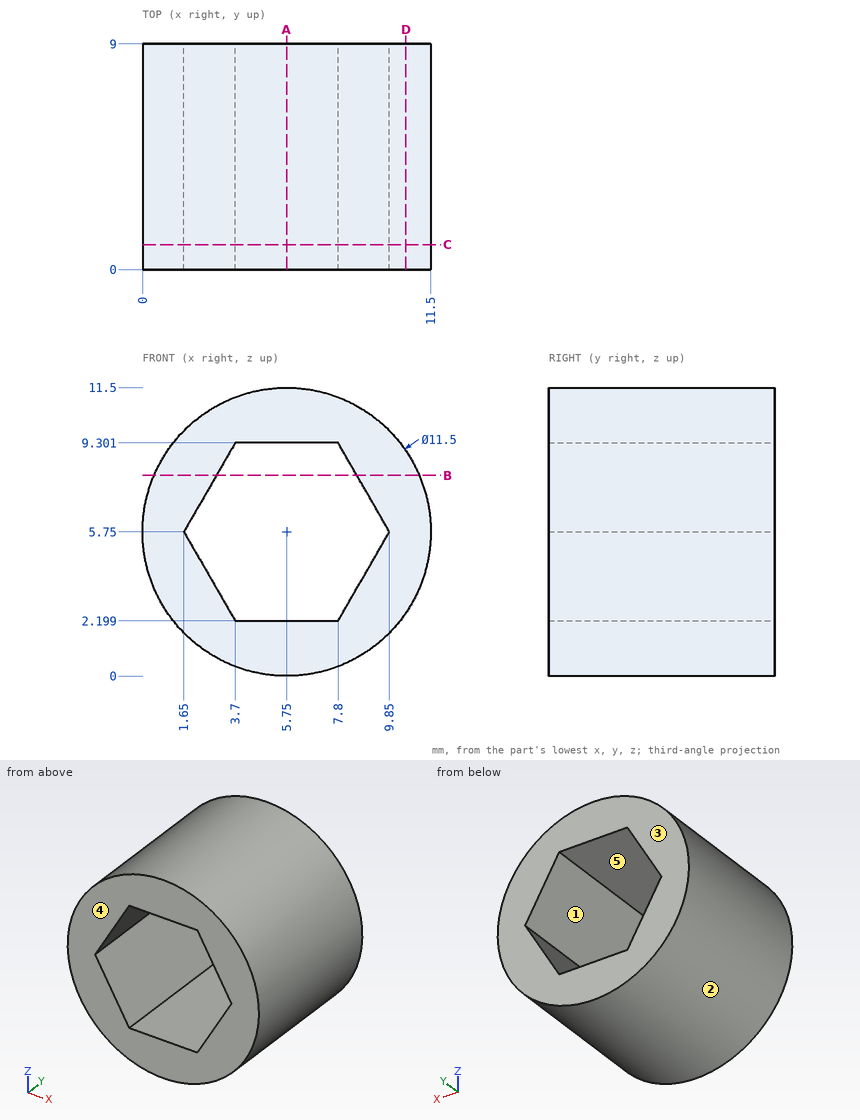
Study the drawing (mm; zero at the part's minimum x, y, z) and answer. A direction names the side the tool comes from. Round coordinates to 2 decimals unless told otherwise and drop trailing zeros. Write each loop counter-clockwise with the first axis right and the second up, starting at its lowest first coordinate (ties: lowest second). Pieces come first, ordered by that corner, then holes.
1) A cutting plane is placed at D-D (x = 10.5). Give the vertices of the cut face in (y, z).
2) Straight lines are drawn through the part: line 1 (Z direction, x = 6, y = 6.25) (1 decimal); line 2 (Z direction, x = 4, y = 4.25); line 3 (X direction, y = 5.5, z = 4.5). For each, find the intervals that lie inside material, in ascending order.
3) Given pin 1 Ø1.2 at (x, y) = (6.5, 2.5) entering from +Z; pin 2 Ø1.2 at (x, y) = (7, 4) entering from -Z; pin 3 Ø1 at (y, z) = (4, 1.5) entering from -X, each flat-ended and moving along its own axis, determine where each tip first touches the part or whether it passes through.
4) A tool of negligible diameter and unlimited length cuts with its end or side. For the marked faces 4 and 5, from which of +Z, -Z, +X, -X, +Y, -Y can it reach the whole face along a straight path? Write none if from no direction.
5) A cutting plane is placed at A-A (x = 5.75). Give the vertices of the cut face in (y, z), plus the area to 3 significant figures.
6) A cutting plane is placed at B-B (z = 8). Give the vertices of the cut face in (x, y).
7) A cutting plane is placed at C-C (y = 1). Give the vertices of the cut face in (x, z), plus the area to 3 significant figures.
8) The mould has two halves that part along Z. Classify the marked faces 1, 2 and 3: pulls with the +Z half, pulls with the -Z half, needs draft (parallel to the pull), parting line crosses it, or undercut.
Completed:
1. outline: (0, 2.51) - (9, 2.51) - (9, 8.99) - (0, 8.99) - close
2. line 1: z = 0 to 2.2, 9.3 to 11.5
2. line 2: z = 0.27 to 2.2, 9.3 to 11.23
2. line 3: x = 0.14 to 2.37, 9.13 to 11.36
3. pin 1: stops at z = 11.5
3. pin 2: stops at z = 0.04
3. pin 3: stops at x = 1.39
4. face 4: +Z, -Z, +X, -X, -Y
4. face 5: +Y, -Y
5. outline: (0, 0) - (9, 0) - (9, 2.2) - (0, 2.2) - close; (0, 9.3) - (9, 9.3) - (9, 11.5) - (0, 11.5) - close
5. area: 39.6 mm2
6. outline: (0.46, 0) - (2.95, 0) - (2.95, 9) - (0.46, 9) - close; (8.55, 0) - (11.04, 0) - (11.04, 9) - (8.55, 9) - close
7. outline: circle Ø11.5 at (5.75, 5.75); hole (1.65, 5.75) - (3.7, 2.2) - (7.8, 2.2) - (9.85, 5.75) - (7.8, 9.3) - (3.7, 9.3) - close
7. area: 60.2 mm2
8. face 1: undercut
8. face 2: parting line crosses it
8. face 3: needs draft
